Input: part model. Units: mm. Frame: model coordinates. Round coordinates to 2 decimals unless told otherwise and drop trailing zeros. Write each loop counter-clockwise with the first axis right and the second up, starting at its lowest first coordinate (ties: lowest second). Pieces come first, ordered by that corner, then holes. Notation, with made-up numbers: (21, 29.25) -> (67, 29.25) arc R24 ccw to (67, 67.25) -> close; hole circle Ø7 at (79.5, 82.25). An arc over 180 degrees is marked (long way). Write item = value, one per line.
Autodesk Inventor part; units mm, degrees
ref_plane "YZ Plane" through (0, 0, 0) normal (1, 0, 0) x (0, 1, 0)
ref_plane "XZ Plane" through (0, 0, 0) normal (0, 1, 0) x (-1, 0, 0)
ref_plane "XY Plane" through (0, 0, 0) normal (0, 0, 1) x (1, 0, 0)
sketch "Sketch1" plane through (0, 0, 0) normal (0, 1, 0) x (-1, 0, 0)
  circle A0 centre (0, 0) radius 2.3
  circle A1 centre (0, 0) radius 10
  circle A2 centre (0, 0) radius 2.1
  dimension "d0" = 0.2
extrude "Extrusion1" add sketch "Sketch1" along normal blind 7.5 contours A0 | A1 | A2
fillet "Fillet1" radius 1 1 edges at (10, 7.5, 0)
extrude "Extrusion2" add sketch "Sketch1" against normal blind 2 contours A2
chamfer "Chamfer1" distance 0.5 angle 45 1 edges at (2.1, -2, 0)
properties part number "knob_top"
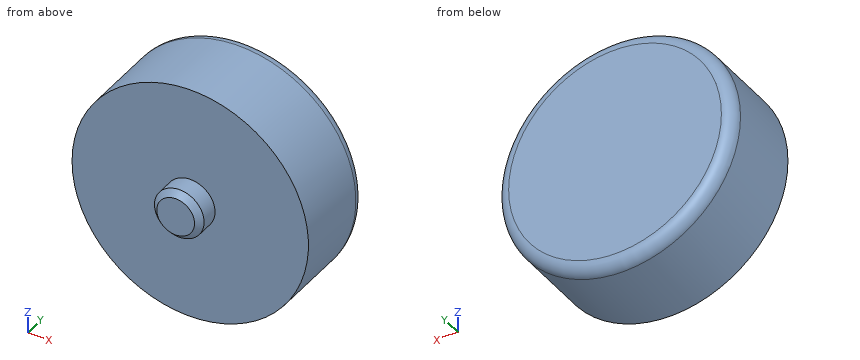
1) Cut plane B-B (x = 0). Return the cut outline in (y, z).
Solutions:
outline = (-2, -1.6) -> (-1.5, -2.1) -> (0, -2.1) -> (0, -10) -> (6.5, -10) arc R1 ccw to (7.5, -9) -> (7.5, 9) arc R1 ccw to (6.5, 10) -> (0, 10) -> (0, 2.1) -> (-1.5, 2.1) -> (-2, 1.6) -> close
2) Cut plane C-C (y = 2.5). Return the cut outline in (x, z), and give its area (3 significant figures).
Solutions:
outline = circle Ø20 at (0, 0)
area = 314 mm^2
3) Line query: L1, parallel to Y at x = -0.25, z = 5; L2, parallel to Z at x = -2, y = 4.75; L3, parallel to Z at x = -6.5, y = 3.75. Output: solid intervals per line, ascending. Write a range as from..to.
Solutions:
L1 = 0..7.5
L2 = -9.8..9.8
L3 = -7.6..7.6
4) First-contact query: P1, Ø2, axis at y = 1.5, z = 2.5, coming from the +X side; P2, Ø4, axis at x = 3, y = 6, coming from the +Z side; P3, Ø2, axis at x = 5, y = 1, coming from the -Z side. Flat tips, straight axial feed; report the tip coordinate or a pass-through.
Solutions:
P1 = 9.89
P2 = 9.95
P3 = -9.17
5) Cut plane A-A (z = 0). Return the cut outline in (x, y).
Solutions:
outline = (-10, 0) -> (-2.1, 0) -> (-2.1, -1.5) -> (-1.6, -2) -> (1.6, -2) -> (2.1, -1.5) -> (2.1, 0) -> (10, 0) -> (10, 6.5) arc R1 ccw to (9, 7.5) -> (-9, 7.5) arc R1 ccw to (-10, 6.5) -> close
6) Cut plane D-D (y = 7.25). Return the cut outline in (x, z), and give its area (3 significant figures).
Solutions:
outline = circle Ø19.32 at (0, 0)
area = 293 mm^2
